Work out the finished part from the listing and answer in its coordinate system (mm). A direction names the side the tool comes from. Coordinates: 2 decimals unless noted, no trailing zeros. Write each loop counter-clockwise with the first axis right and the second up, starting at its lowest first coordinate (ties: lowest second). Pieces come first, ordered by that corner, then holes. Notation, with made-up numbers: M -33,65.25 L 3,65.25 A28 cw 3,86.25 Z; hole C 74,-8.5 d10. An arc over 180 degrees is marked long. Use CSV: the item, a comma, the result in double quotes.
from build123d import *

# Parameters (mm, degrees)
BOSS_EXTRUDE1_DEPTH = 5
SKETCH3_W           = 8
SKETCH3_H           = 4
BOSS_EXTRUDE2_DEPTH = 3
FILLET1_START       = -3.841593316
FILLET1_DEPTH       = 8
CUT_EXTRUDE1_START  = -10
CUT_EXTRUDE1_DEPTH  = 10
FILLET2_R           = 3
SKETCH6_R           = 1.25
CUT_EXTRUDE2_DEPTH  = 5
CUT_EXTRUDE3_START  = -5
SKETCH7_R           = 1.25
CUT_EXTRUDE3_DEPTH  = 5


with BuildPart() as part:
    # Sketch1 → Boss-Extrude1 (new body)
    with BuildSketch(Plane(origin=(0, 0, 0), x_dir=(1, 0, 0), z_dir=(0, 1, 0))):
        with BuildLine():
            Line((-30, 0), (30, 0))
            ThreePointArc((30, 0), (0, 30), (-30, 0))
        make_face()
    extrude(amount=BOSS_EXTRUDE1_DEPTH)

    # Sketch3 → Boss-Extrude2 (add)
    with BuildSketch(Plane(origin=(0, 5, 0), x_dir=(1, 0, 0), z_dir=(0, 1, 0))):
        with Locations((0.158406684, 24.731666579)):
            Rectangle(SKETCH3_W, SKETCH3_H)
    extrude(amount=BOSS_EXTRUDE2_DEPTH)

    # Fillet1: read off the stored shape, not the designer's step
    # Fillet1 outline → Fillet1 (cut)
    with BuildSketch(Plane.YZ.offset(FILLET1_START)):
        with BuildLine():
            Line((8, -22.731666579), (5, -22.731666579))
            add(Edge.make_bspline(
                [(5, -22.731666579), (8, -23.506263249), (8, -26.604649926)],
                knots=[0, 0, 0, 1, 1, 1], degree=2, weights=[1, 0.057495957, 1]))
            Line((8, -26.604649926), (8, -22.731666579))
        make_face()
    extrude(amount=FILLET1_DEPTH, mode=Mode.SUBTRACT)

    # Sketch5 → Cut-Extrude1 (cut)
    with BuildSketch(Plane(origin=(0, 5, 0), x_dir=(1, 0, 0), z_dir=(0, 1, 0)).offset(CUT_EXTRUDE1_START)):
        with BuildLine():
            Line((-22.580398915, 0), (-22.580398915, 5))
            Line((-22.580398915, 5), (-29.580398915, 5))
            ThreePointArc((-29.580398915, 5), (-29.894915684, 2.508787808), (-30, 0))
            Line((-30, 0), (-22.580398915, 0))
        make_face()
        with BuildLine():
            Line((22.580398915, 5), (29.580398915, 5))
            ThreePointArc((29.580398915, 5), (29.894915684, 2.508787808), (30, 0))
            Line((30, 0), (22.580398915, 0))
            Line((22.580398915, 0), (22.580398915, 5))
        make_face()
    extrude(amount=CUT_EXTRUDE1_DEPTH, mode=Mode.SUBTRACT)

    # Fillet2
    fillet2_edges = [part.edges().sort_by_distance(p)[0] for p in [
        (0, 5, 0),
    ]]
    fillet(fillet2_edges, radius=FILLET2_R)

    # Sketch6 → Cut-Extrude2 (cut)
    with BuildSketch(Plane(origin=(22.580398915, 0, 0), x_dir=(0, 0, -1), z_dir=(1, 0, 0))):
        with Locations((3, 2.25)):
            Circle(SKETCH6_R)
    extrude(amount=-CUT_EXTRUDE2_DEPTH, mode=Mode.SUBTRACT)

    # Sketch7 → Cut-Extrude3 (cut)
    with BuildSketch(Plane.ZY.offset(22.580398915).offset(CUT_EXTRUDE3_START)):
        with Locations(Location((-3, 2.25, 0), (0, 0, 180))):
            Circle(SKETCH7_R)
    extrude(amount=CUT_EXTRUDE3_DEPTH, mode=Mode.SUBTRACT)


solid = part.part
Item 1: The part is cut by section A-A (x = 9.5). Write down the section's boundary in (y, z).
Answer:
outline,"M 0,-28.46 L 5,-28.46 L 5,-3 A3 ccw 2,0 L 0,0 Z"
Item 2: The part is cut by section B-B (z = -20.75). Write down the section's boundary in (x, y), then the cut area to 3 significant figures.
Answer:
outline,"M -21.67,0 L 21.67,0 L 21.67,5 L -21.67,5 Z"
area,"217 mm2"
Item 3: Consider probe 1 along Y at (x, z) = (-19, -11); probe 2 along X at (y, z) = (1.5, -19.75); probe 3 along Z at (x, y) = (-19.85, 2.25). Determine where each line is inside the solid, lowest interval first.
Answer:
probe 1,"y = 0 to 5"
probe 2,"x = -22.58 to 22.58"
probe 3,"z = -22.49 to -4.25, -1.75 to -0.01"
Item 4: The part is cut by section C-C (x = -14.5). Write down the section's boundary in (y, z), then the cut area to 3 significant figures.
Answer:
outline,"M 0,-26.26 L 5,-26.26 L 5,-3 A3 ccw 2,0 L 0,0 Z"
area,"129 mm2"
Item 5: For a pull along Z with two mould halves and no side action, classify faces 1 (the face through (22.58, 2, -1)), 2 (the face through (0.32, 4.1, -0.86)), 3 (the face through (20, 3, -4)), 4 (the face through (-17.58, 2, -3)) as released by +Z, released by -Z, zero draft, split by the parting line, or undercut.
Answer:
face 1,"zero draft"
face 2,"released by +Z"
face 3,"undercut"
face 4,"undercut"
Item 6: A tool of negligible diameter and unlimited length cuts with its end or side. For faces 5 (the face through (17.58, 2, -3)), 6 (the face through (-3.842, 6, -25)), 7 (the face through (26, 2, -5)), 8 (the face through (-20, 1.9, -4.2)), from which of +Z, -Z, +X, -X, +Y, -Y can it reach the whole face along a straight path? Write none if from no direction.
Answer:
face 5,"+X"
face 6,"+Z, -Z, -X, +Y"
face 7,"+Z, +X, +Y, -Y"
face 8,"-X"
Item 7: Given pin 1 (5 mm diameter, centred on x = -8, z = -4.5, fed in from +Y); pin 2 (1.5 mm diameter, centred on y = 6, z = -24, fed in from +X); pin 3 (2 mm diameter, centred on y = 3.5, z = -10.5, fed in from +X); pin 4 (1.5 mm diameter, centred on x = 21, z = -24, fed in from -Y), each flat-ended and moving along its own axis, determine where each tip first touches the part or whether it passes through.
Answer:
pin 1,"stops at y = 5"
pin 2,"stops at x = 4.16"
pin 3,"stops at x = 28.46"
pin 4,"passes through"
